```python
from build123d import *

# Parameters (mm, degrees)
SKETCH23_W          = 85
SKETCH23_H          = 85
BOSS_EXTRUDE1_DEPTH = 7
SKETCH26_R          = 49
SKETCH26_R_2        = 40.588103662
BOSS_EXTRUDE2_DEPTH = 20
SKETCH28_R          = 36
CUT_EXTRUDE5_DEPTH  = 84.731714422
SKETCH29_R          = 2.75
CUT_EXTRUDE6_DEPTH  = 7
FILLET1_R           = 5
FILLET2_R           = 5


# Read off the part's stored shape, not the designer's step: Loft-Thin1
with BuildPart() as part:
    # Loft-Thin1 outline → Loft-Thin1 (revolve)
    with BuildSketch(Plane.YX):
        Polygon((34.088103662, 20), (40.588103662, 0), (49, 0), (42.5, 20), align=None)
    revolve(axis=Axis((0, 0, 0), (1, 0, 0)))

    # Sketch23 → Boss-Extrude1 (add)
    with BuildSketch(Plane(origin=(20, 0, 0), x_dir=(0, 0, -1), z_dir=(1, 0, 0))):
        Rectangle(SKETCH23_W, SKETCH23_H)
    extrude(amount=BOSS_EXTRUDE1_DEPTH)

    # Sketch26 → Boss-Extrude2 (add)
    with BuildSketch(Plane.ZY):
        with Locations(Location((0, 0, 0), (0, 0, 180))):
            Circle(SKETCH26_R)
        with Locations(Location((0, 0, 0), (0, 0, 180))):
            Circle(SKETCH26_R_2, mode=Mode.SUBTRACT)
    extrude(amount=BOSS_EXTRUDE2_DEPTH)

    # Sketch28 → Cut-Extrude5 (cut, through all)
    with BuildSketch(Plane(origin=(27, 0, 0), x_dir=(0, 0, -1), z_dir=(1, 0, 0))):
        Circle(SKETCH28_R)
    extrude(amount=-CUT_EXTRUDE5_DEPTH, mode=Mode.SUBTRACT)

    # Sketch29 → Cut-Extrude6 (cut)
    with BuildSketch(Plane(origin=(27, 0, 0), x_dir=(0, 0, -1), z_dir=(1, 0, 0))):
        with Locations((-35.5, 35.5)):
            Circle(SKETCH29_R)
        with Locations(Location((35.5, 35.5, 0), (0, 0, 180))):
            Circle(SKETCH29_R)
        with Locations(Location((-35.5, -35.5, 0), (0, 0, 180))):
            Circle(SKETCH29_R)
        with Locations((35.5, -35.5)):
            Circle(SKETCH29_R)
    extrude(amount=-CUT_EXTRUDE6_DEPTH, mode=Mode.SUBTRACT)

    # Fillet1
    fillet1_edges = [part.edges().sort_by_distance(p)[0] for p in [
        (23.5, -42.5, -42.5),
    ]]
    fillet(fillet1_edges, radius=FILLET1_R)

    # Fillet2
    fillet2_edges = [part.edges().sort_by_distance(p)[0] for p in [
        (23.5, -42.5, 42.5),
        (23.5, 42.5, 42.5),
        (23.5, 42.5, -42.5),
    ]]
    fillet(fillet2_edges, radius=FILLET2_R)


solid = part.part
```
Here's how the part is built. I have some questions about the finished solid (model axes, mm). A direction names the side the tool comes from. Round coordinates to 2 decimals unless told otherwise and drop trailing zeros. Order: outer loops, then holes, each group sorted by start corner. A loop starts at its lowest first (then second) coordinate and runs counter-clockwise, first axis right, second up. Notation, with made-up numbers: (-32.75, 78) -> (-13.75, 78) arc R15 cw to (-13.75, 83) -> close; hole circle Ø8 at (35, 89.25). An arc over 180 degrees is marked (long way). Use a Markdown table: item, result. Add a question column.
(1) If we mould it in two halves opening along Y, with no side actions, what happens to faces 1 (the face through (23.55, 41, -41.07)), 2 (the face through (23.549, 37.359, 37.527)), 3 (the face through (19.03, -5.57, 42.45))? For each: released by +Y, released by -Y, zero draft, split by the parting line, or undercut.
(2) For faces 4 (the face through (23.549, 33.641, -37.527)), 5 (the face through (20, -32, -32)), 6 (the face through (23, 42.5, 1)), 7 (the face through (23, -1, 42.5)), 8 (the face through (23, -1, -42.5)), which set-ups out of +Z, -Z, +X, -X, +Y, -Y let a thin tool reach every point of the face, with its end or its side?
(3) For pin 1 Ø12.5 at (y, z) = (15, -20.5) entering from -X; pin 2 Ø3 at (x, z) = (-12, 31.5) entering from +Y; pin 3 Ø2 at (x, z) = (-0.5, -17) entering from +Y; pin 4 Ø2 at (x, z) = (7.5, -30) entering from -Y, each with a flat end and sliding along its axis, tell me the tip position at first contact or that it passes through.
(4) Suppose I cut it at A-A, the plane x = -7. Please give me the cut outline in (y, z), and give its area (3 significant figures).
(5) I need wall thicknesses on line 1 along Z through (x, y) = (23, 0); line 2 along Z through (x, y) = (22, 4.5). Which ranges of each line are inside material? Lowest first, please.
Verdict:
| question | item | result |
|---|---|---|
| 1 | face 1 | released by +Y |
| 1 | face 2 | undercut |
| 1 | face 3 | split by the parting line |
| 2 | face 4 | +X |
| 2 | face 5 | -Z, -Y |
| 2 | face 6 | +Z, -Z, +X, +Y |
| 2 | face 7 | +Z, +X, +Y, -Y |
| 2 | face 8 | -Z, +X, +Y, -Y |
| 3 | pin 1 | through |
| 3 | pin 2 | y = 38.74 |
| 3 | pin 3 | y = 46.31 |
| 3 | pin 4 | y = -36.53 |
| 4 | outline | circle Ø98 at (0, 0); hole circle Ø81.18 at (0, 0) |
| 4 | area | 2,370 mm2 |
| 5 | line 1 | -42.5 to -36, 36 to 42.5 |
| 5 | line 2 | -42.5 to -35.72, 35.72 to 42.5 |
